Source: CAD feature listing. Evaluate the final solid. Frame: model axes, mm. Give positions to 0.01 mm unless a question says otherwise; leave off trailing zeros. Write each loop counter-clockwise with the first axis right and the second up, starting at its lowest first coordinate (ties: lowest second). Pieces come first, ordered by that corner, then holes. Notation, with made-up numbers: (-20.75, 37.5) -> (18.25, 37.5) arc R22 cw to (18.25, 43.5) -> close; hole circle Ø5 at (6.25, -29.5). An arc over 180 degrees is marked (long way). Use one line per item in the form item = value. Start each with the question number.
(1) Material intervals for line 1 along Y through (x, z) = (0.25, 0); line 2 along Z through (x, y) = (1, -11.5) (3 decimals); line 3 along Z through (x, y) = (-1.75, 0.5), sorted ascending. Write a range as from..to.
(2) Cut plane B-B, the plane y = -21.59. Output: boundary loops of the cut face in (x, z) (3 decimals).
(3) Cut plane D-D, the plane z = -20. Output: boundary loops of the cut face in (x, y) (3 decimals).
(4) Cut plane C-C, the plane z = 8. Output: boundary loops of the cut face in (x, y) (3 decimals).
(5) First-contact query: P1, Ø1.5, axis at x = 0.5, z = 32, coming from the -Y side (3 decimals); P2, Ø2, axis at x = 0, z = 21, coming from the -Y side; P3, Ø3, axis at x = -1.5, z = 30.5, coming from the +Y side (3 decimals). Flat tips, straight axial feed; report the tip coordinate or a pass-through.
(6) Cut plane A-A, the plane x = 0. Count the separate pieces of the cut face and the enclosed holes in it, and give its area (3 significant figures).
from build123d import *

# Parameters (mm, degrees)
BOSS_EXTRUDE1_DEPTH     = 3.175
SKETCH15_W              = 6.35
SKETCH15_H              = 19.05
CUT_EXTRUDE4_DEPTH      = 4.175
CUT_EXTRUDE4_DEPTH_BACK = 4.175
SKETCH37_R              = 1.5
SKETCH37_R_2            = 4.7625
CUT_EXTRUDE15_DEPTH     = 7.35
SKETCH47_R              = 1.27
CUT_EXTRUDE18_DEPTH     = 7.35
FILLET14_R              = 1.27
FILLET15_R              = 1.27


with BuildPart() as part:
    # Sketch5 → Boss-Extrude1 (new body, symmetric)
    with BuildSketch(Plane(origin=(0, 0, 0), x_dir=(0, 0, -1), z_dir=(1, 0, 0))):
        with BuildLine():
            Line((19.05, -23.926477372), (19.05, 0))
            ThreePointArc((19.05, 0), (17.582566657, 7.331838088), (13.406341233, 13.534124085))
            Line((13.406341233, 13.534124085), (-10.465609794, 37.180687347))
            ThreePointArc((-10.465609794, 37.180687347), (-13.921973015, 37.855427776), (-15.875, 34.925))
            Line((-15.875, 34.925), (-15.875, 3.175))
            Line((-15.875, 3.175), (-50.8, 3.175))
            Line((-50.8, 3.175), (-50.8, -28.575))
            Line((-50.8, -28.575), (-28.575, -28.575))
            Line((-28.575, -28.575), (25.4, -34.925))
            Line((25.4, -34.925), (38.1, -34.925))
            Line((38.1, -34.925), (19.05, -23.926477372))
        make_face()
    extrude(amount=BOSS_EXTRUDE1_DEPTH, both=True)

    # Sketch15 → Cut-Extrude4 (cut, two sides)
    with BuildSketch(Plane(origin=(0, 0, 0), x_dir=(0, 0, -1), z_dir=(1, 0, 0))) as cut_extrude4_sk:
        with Locations((-38.1, -19.05)):
            Rectangle(SKETCH15_W, SKETCH15_H)
    extrude(amount=CUT_EXTRUDE4_DEPTH, mode=Mode.SUBTRACT)
    extrude(cut_extrude4_sk.sketch, amount=-CUT_EXTRUDE4_DEPTH_BACK, mode=Mode.SUBTRACT)

    # Sketch37 → Cut-Extrude15 (cut, through all)
    with BuildSketch(Plane(origin=(3.175, 0, 0), x_dir=(0, 0, -1), z_dir=(1, 0, 0))):
        with Locations((0, -9.5)):
            Circle(SKETCH37_R)
        with Locations((0, 9.5)):
            Circle(SKETCH37_R)
        with Locations((8, 0)):
            Circle(SKETCH37_R)
        with Locations((-8, 0)):
            Circle(SKETCH37_R)
        Circle(SKETCH37_R_2)
    extrude(amount=-CUT_EXTRUDE15_DEPTH, mode=Mode.SUBTRACT)

    # Sketch47 → Cut-Extrude18 (cut, through all)
    with BuildSketch(Plane.ZY.offset(3.175)):
        with Locations((14.14272, -21.59)):
            Circle(SKETCH47_R)
    extrude(amount=-CUT_EXTRUDE18_DEPTH, mode=Mode.SUBTRACT)

    # Fillet14
    fillet14_edges = [part.edges().sort_by_distance(p)[0] for p in [
        (0, -34.925, -38.1),
    ]]
    fillet(fillet14_edges, radius=FILLET14_R)

    # Fillet15
    fillet15_edges = [part.edges().sort_by_distance(p)[0] for p in [
        (0, -28.575, 50.8),
        (0, 3.175, 50.8),
        (0, 3.175, 15.875),
        (0, -28.575, 34.925),
        (0, -28.575, 41.275),
    ]]
    fillet(fillet15_edges, radius=FILLET15_R)


solid = part.part
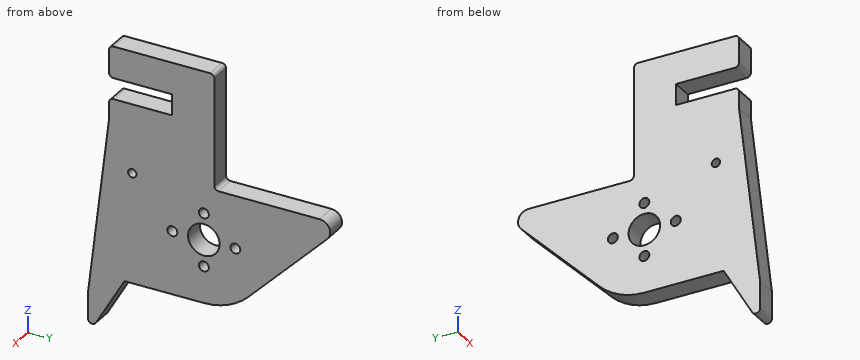
Geometry says:
q1.line_1 = -31.94..-11, -8..-4.76, 4.76..8, 11..26.81
q1.line_2 = -19.05..34.925, 41.275..50.8
q1.line_3 = -19.04..-9.41, -6.59..-4.74, 4.74..6.59, 9.41..50.8
q2.outline = (-3.175, -19.05) -> (3.175, -19.05) -> (3.175, 12.873) -> (-3.175, 12.873) -> close; (-3.175, 15.413) -> (3.175, 15.413) -> (3.175, 34.925) -> (-3.175, 34.925) -> close; (-3.175, 41.275) -> (3.175, 41.275) -> (3.175, 50.8) -> (-3.175, 50.8) -> close
q3.outline = (-3.175, -34.29) -> (3.175, -34.29) -> (3.175, -24.475) -> (-3.175, -24.475) -> close
q4.outline = (-3.175, -30.996) -> (3.175, -30.996) -> (3.175, -1.5) -> (-3.175, -1.5) -> close; (-3.175, 1.5) -> (3.175, 1.5) -> (3.175, 34.738) -> (-3.175, 34.738) -> close
q5.P1 = -28.575
q5.P2 = -29.58
q5.P3 = 3.175
q6.separate_pieces = 1
q6.enclosed_holes = 6
q6.area = 2,970 mm^2
